Part model, mm, in its own coordinate system. Face numbers are marked on the shaded views. Round coordinates to 2 decimals unless told otherwise and drop trailing zeros. Loops run counter-clockwise (first coordinate to the right, second up) from the corner with the lowest first, then second, coordinate; pieces in that order, holes last.
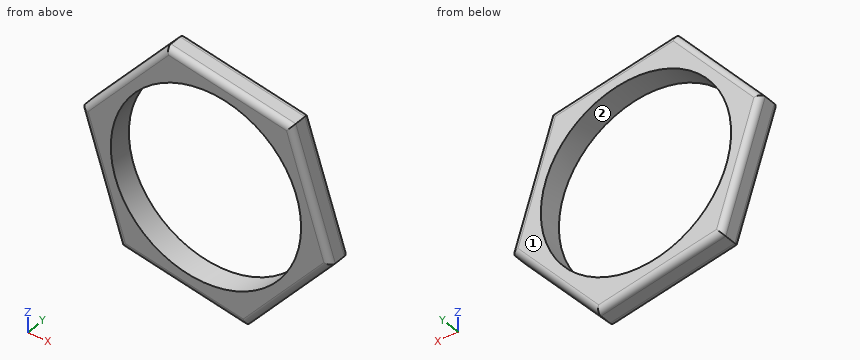
from build123d import *

# Parameters (mm, degrees)
SKETCH_1_R      = 15.5
EXTRUDE_1_DEPTH = 4
FILLET_1_R      = 1


with BuildPart() as part:
    # 草图1 → 凸台-拉伸1 (new body)
    with BuildSketch(Plane(origin=(0, 0, 0), x_dir=(1, 0, 0), z_dir=(0, 1, 0))):
        Polygon((13.894572462, -15.457711864), (20.33405739, 4.304196795), (6.439484928, 19.761908659), (-13.894572462, 15.457711864), (-20.33405739, -4.304196795), (-6.439484928, -19.761908659), align=None)
        Circle(SKETCH_1_R, mode=Mode.SUBTRACT)
    extrude(amount=EXTRUDE_1_DEPTH)

    # 圆角1
    fillet_1_edges = [part.edges().sort_by_distance(p)[0] for p in [
        (13.386771159, 4, -12.033052727),
        (-3.727543767, 4, -17.609810262),
        (-17.114314926, 4, -5.576757535),
        (-13.386771159, 4, 12.033052727),
        (3.727543767, 4, 17.609810262),
        (-13.386771159, 0, 12.033052727),
        (-17.114314926, 0, -5.576757535),
        (-3.727543767, 0, -17.609810262),
        (17.114314926, 4, 5.576757535),
        (13.386771159, 0, -12.033052727),
        (17.114314926, 0, 5.576757535),
        (3.727543767, 0, 17.609810262),
    ]]
    fillet(fillet_1_edges, radius=FILLET_1_R)


solid = part.part
1) Slice it at A-A, the plane y = 2.1. Give the cut face in (x, z).
Values:
outline: (-20.33, 4.3) - (-13.89, -15.46) - (6.44, -19.76) - (20.33, -4.3) - (13.89, 15.46) - (-6.44, 19.76) - close; hole circle Ø31 at (0, 0)
2) Wall check: line 1 along X through (y, z) = (1.2, -12); line 2 along X through (y, z) = (1.55, -6.5); line 3 along Z through (x, y) = (13.5, 3.3). Give the ranges that are in metal, low to high.
Values:
line 1: x = -15.02 to -9.81, 9.81 to 13.42
line 2: x = -16.81 to -14.07, 14.07 to 18.36
line 3: z = -11.84 to -7.62, 7.62 to 15.49
3) Mould opens along Z. For the marked faces 1 and 2 say: released by +Z, released by -Z, zero draft, split by the parting line, or undercut.
Values:
face 1: zero draft
face 2: undercut
4) Drop a flat-ended pin along its axis: pin 1 Ø1.5 at (x, y) = (2.5, 3.5) entering from +Z. Give the stop position or say it passes through.
Values:
pin 1: stops at z = 18
